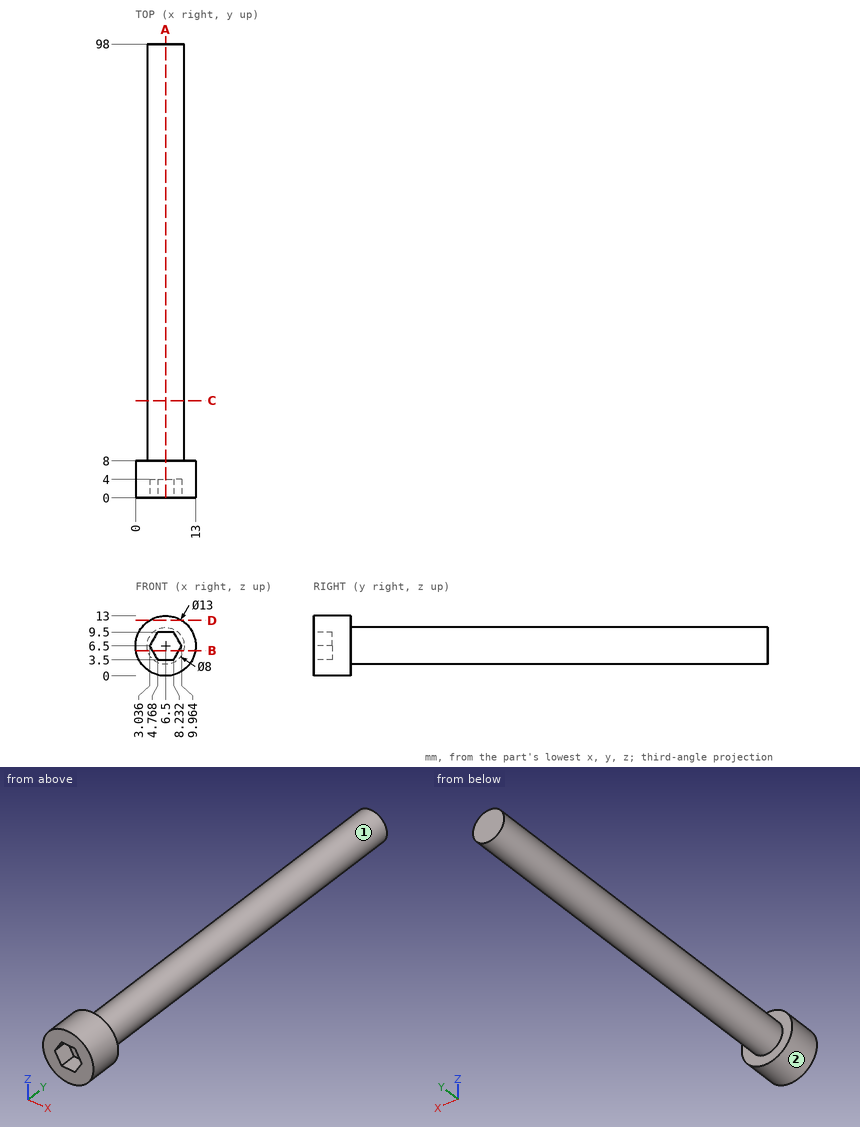
Check sheet for the drawn part. Datum: minimum x, y, z corner. Units: mm. A direction names the side the tool comes from. Coordinates: 2 decimals unless noted, no trailing zeros. Loops run counter-clockwise (first coordinate to the right, second up) from the corner with the lowest first, then second, coordinate; pieces in that order, holes last. Notation, with made-up numbers: (41.5, 84.5) - (73.5, 84.5) arc R34 ccw to (73.5, 121.5) - close; hole circle Ø4 at (55, 79.5). An arc over 180 degrees is marked (long way). Put each result on its own line as item: value.
Item 1: Set-up check for the marked faces 1 and 2: record each of +Z, -Z, +X, -X, +Y, -Y from which the full face is reachable in a straight line by a thin tool's end or side.
Conclusion:
face 1: +Y
face 2: +Y, -Y
Item 2: Gauge pin test, flat ends, axial feed: pin 1 Ø3 at (x, y) = (4.5, 78.5) entering from -Z; pin 2 Ø2 at (y, z) = (43, 8) entering from -X; pin 3 Ø2 at (y, z) = (34, 10.5) entering from +X. Record the tip position at first contact, or that the pin passes through.
Conclusion:
pin 1: stops at z = 2.53
pin 2: stops at x = 2.53
pin 3: stops at x = 9.15
Item 3: Section check D-D (z = 12). Enter the section's corners in (x, y), then the cut area to 3 significant figures.
Conclusion:
outline: (3.04, 0) - (9.96, 0) - (9.96, 8) - (3.04, 8) - close
area: 55.4 mm2
Item 4: Section check B-B (z = 5.5). Enter the section's corners in (x, y).
Conclusion:
outline: (0.08, 0) - (3.61, 0) - (3.61, 4) - (9.39, 4) - (9.39, 0) - (12.92, 0) - (12.92, 8) - (10.37, 8) - (10.37, 98) - (2.63, 98) - (2.63, 8) - (0.08, 8) - close
Item 5: Section check A-A (x = 6.5). Enter the section's corners in (y, z), then the cut area to 3 significant figures.
Conclusion:
outline: (0, 0) - (8, 0) - (8, 2.5) - (98, 2.5) - (98, 10.5) - (8, 10.5) - (8, 13) - (0, 13) - (0, 9.5) - (4, 9.5) - (4, 3.5) - (0, 3.5) - close
area: 800 mm2
Item 6: Scan lines: line 1 along Y through (x, z) = (7.5, 4); line 2 along X through (y, z) = (76.5, 8.5); line 3 along X through (y, z) = (38, 6.5). Record each from-to range of solid material in increasing order.
Conclusion:
line 1: y = 4 to 98
line 2: x = 3.04 to 9.96
line 3: x = 2.5 to 10.5
Item 7: Section check C-C (y = 21). Enter the section's corners in (x, z), then the cut area to 3 significant figures.
Conclusion:
outline: circle Ø8 at (6.5, 6.5)
area: 50.3 mm2
